The model under review builds one solid part; all positions refer to its coordinate system, in mm. A direction names the side the tool comes from. Coordinates: 2 decimals unless noted, no trailing zeros. Order: outer loops, then holes, each group sorted by start corner. A loop starts at its lowest first (then second) coordinate and runs counter-clockwise, first axis right, second up.
```python
from build123d import *

# Parameters (mm, degrees)
F0_W     = 13.0302
F0_H     = 22.352
F1_DEPTH = 263.525
F2_W     = 11.3284
F2_H     = 2.032
F3_DEPTH = 263.526
F4_W     = 9.8552
F4_H     = 13.081
F5_DEPTH = 263.526
F6_W     = 263.525
F6_H     = 2.159
F7_DEPTH = 4.699


with BuildPart() as f1:
    # F0 (on Front) → F1 (new body)
    with BuildSketch(Plane.XZ):
        Rectangle(F0_W, F0_H)
    extrude(amount=F1_DEPTH)

    # F2 (on face) → F3 (cut, through all)
    with BuildSketch(Plane.XZ.offset(263.525)):
        with Locations((0.8509, 7.62)):
            Rectangle(F2_W, F2_H)
    extrude(amount=-F3_DEPTH, mode=Mode.SUBTRACT)

    # F4 (on face) → F5 (cut, through all)
    with BuildSketch(Plane.XZ.offset(263.525)):
        with Locations((1.5875, -2.4765)):
            Rectangle(F4_W, F4_H)
    extrude(amount=-F5_DEPTH, mode=Mode.SUBTRACT)

    # F6 (on face) → F7 (cut)
    with BuildSketch(Plane.YZ.offset(6.5151)):
        with Locations((-131.7625, -10.0965)):
            Rectangle(F6_W, F6_H)
    extrude(amount=-F7_DEPTH, mode=Mode.SUBTRACT)


solid = f1.part
```
(1) We need section C-C, the plane z = 0. Write out the cut boundary in (x, y) (3 decimals).
A:
outline: (-6.515, -263.525) - (-3.34, -263.525) - (-3.34, 0) - (-6.515, 0) - close
(2) We need section A-A, the plane x = -0.75. Write out the cut boundary in (y, z) (3 decimals), and give its area (3 significant figures).
A:
outline: (-263.525, -11.176) - (0, -11.176) - (0, -9.017) - (-263.525, -9.017) - close; (-263.525, 4.064) - (0, 4.064) - (0, 6.604) - (-263.525, 6.604) - close; (-263.525, 8.636) - (0, 8.636) - (0, 11.176) - (-263.525, 11.176) - close
area: 1,910 mm2
(3) For pin 1 Ø2.5 at (y, z) = (-114.5, -10.5) entering from +X; pin 2 Ø2 at (x, y) = (5, -178) entering from -Z; pin 3 Ø4 at (y, z) = (-191.5, -3) entering from +X, all flat-tipped, find the tip position at first contact; note any pin that passes through.
A:
pin 1: stops at x = 1.82
pin 2: stops at z = 4.06
pin 3: stops at x = -3.34
(4) Draft analysis for pull direction Z (two halves, no side actions). For faces 3 (the face through (0, -130, 11.176)), 4 (the face through (-4, 0, 3)), 5 (the face through (1, -134, 6.604)), 6 (the face through (-2, -130, -11.176)), state which applies: released by +Z, released by -Z, zero draft, split by the parting line, or undercut.
A:
face 3: released by +Z
face 4: zero draft
face 5: undercut
face 6: released by -Z
(5) Machinability: for faces 1 (the face through (-6.515, -130, 0)), 2 (the face through (1, -134, 8.636)), which of the approach directions +Z, -Z, +X, -X, +Y, -Y give a long, thin tool a straight path to every point of the face, cutting with its end or side? Answer none if there is none.
A:
face 1: +Z, -Z, -X, +Y, -Y
face 2: +X, +Y, -Y
(6) Wall thickness on probe 1 along Z at (x, y) = (1.25, -184); probe 2 along Z at (x, y) = (-4, -108); probe 3 along Z at (x, y) = (3, -103.5): over which ranges is each line inside the solid? List them lowest first.
A:
probe 1: z = -11.18 to -9.02, 4.06 to 6.6, 8.64 to 11.18
probe 2: z = -11.18 to 6.6, 8.64 to 11.18
probe 3: z = 4.06 to 6.6, 8.64 to 11.18
(7) We need section B-B, the plane y = -142. Write out the cut boundary in (x, z), and give its area (3 significant figures).
A:
outline: (-6.52, -11.18) - (1.82, -11.18) - (1.82, -9.02) - (-3.34, -9.02) - (-3.34, 4.06) - (6.52, 4.06) - (6.52, 6.6) - (-4.81, 6.6) - (-4.81, 8.64) - (6.52, 8.64) - (6.52, 11.18) - (-6.52, 11.18) - close
area: 129 mm2
